```python
from build123d import *

# Parameters (mm, degrees)
SKETCH_1_W               = 40
SKETCH_1_H               = 65
SKETCH_1_R               = 12.5
EXTRUDE_1_DEPTH          = 2
CUT_EXTRUDE_1_DEPTH      = 39.369910086
CUT_EXTRUDE_1_DEPTH_BACK = 39.369910086
SKETCH_2_R               = 2.1
CHAMFER_2_SIZE           = 5


with BuildPart() as part:
    # 草图1 → 凸台-拉伸1 (new, symmetric)
    with BuildSketch(Plane.XY):
        Rectangle(SKETCH_1_W, SKETCH_1_H)
        Circle(SKETCH_1_R, mode=Mode.SUBTRACT)
    extrude(amount=EXTRUDE_1_DEPTH, both=True)

    # 草图2 → 切除-拉伸1 (cut, two sides: drawn at the far end of the back side and taken through both)
    with BuildSketch(Plane(origin=(0, 0, -2), x_dir=(-1, 0, 0), z_dir=(0, 0, -1)).offset(-CUT_EXTRUDE_1_DEPTH_BACK)):
        with Locations((-10, 22.5)):
            Circle(SKETCH_2_R)
        with Locations((10, 22.5)):
            Circle(SKETCH_2_R)
        with Locations((10, -22.5)):
            Circle(SKETCH_2_R)
        with Locations((-10, -22.5)):
            Circle(SKETCH_2_R)
    extrude(amount=CUT_EXTRUDE_1_DEPTH + CUT_EXTRUDE_1_DEPTH_BACK, mode=Mode.SUBTRACT)

    # 倒角2
    chamfer_2_edges = [part.edges().sort_by_distance(p)[0] for p in [
        (-20, 32.5, 0),
        (20, 32.5, 0),
        (20, -32.5, 0),
        (-20, -32.5, 0),
    ]]
    chamfer(chamfer_2_edges, length=CHAMFER_2_SIZE)


solid = part.part
```
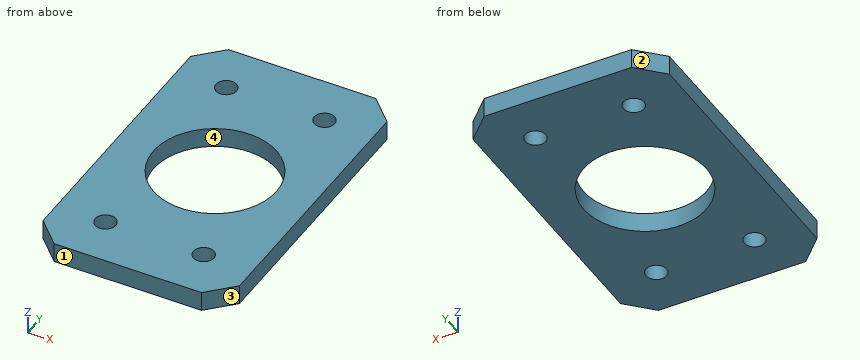
The model under review builds one solid part; all positions refer to its coordinate system, in mm. Face numbers are marked on the shaded views. Coordinates: 2 decimals unless noted, no trailing zeros. Write each loop counter-clockwise with the first axis right and the second up, starting at its lowest first coordinate (ties: lowest second). Pieces come first, ordered by that corner, then holes. Notation, with made-up numbers: (2.5, 75.5) - (54.5, 75.5) arc R30 ccw to (54.5, 100.5) - close; hole circle Ø6 at (33, 25). An arc over 180 degrees is marked (long way). Answer in a Markdown table with one row per item. Add a question column.
Q1. To check wall thickness, follow line 1 along X through (y, z) = (22.5, -0.5); line 2 along Y through (x, z) = (0, -0.95); line 3 along Y through (x, z) = (10, -0.15). State the ranges of each line that lie inside material, in increasing order. Write a range as from..to.
Q2. Consider section B-B on y = -22.5. Give the boundary of the cut face in (x, z), then the cut area to 3 significant figures.
Q3. Clearance check with a flat-ended pin moving along its axis: pin 1 (2.5 mm diameter, centred on x = 10, y = 22.5, fed in from -Z). State where the tip first meets the part, or that it passes through.
Q4. Consider section C-C on x = 0. Give the boundary of the cut face in (y, z), then the cut area to 3 significant figures.
Q5. Consider section D-D on y = 0. Give the boundary of the cut face in (x, z), then the cut area to 3 significant figures.
Q6. Draft analysis for pull direction X (two halves, no side actions). For the marked faces 1, 2, 3 and 4, state which applies: +X half, -X half, draft (parallel to the pull), parting line (faces both ways), or undercut.
Q7. Consider section A-A on x = 10. Give the boundary of the cut face in (y, z).
Answers below:
| question | item | result |
|---|---|---|
| 1 | line 1 | -20..-12.1, -7.9..7.9, 12.1..20 |
| 1 | line 2 | -32.5..-12.5, 12.5..32.5 |
| 1 | line 3 | -32.5..-24.6, -20.4..-7.5, 7.5..20.4, 24.6..32.5 |
| 2 | outline | (-20, -2) - (-12.1, -2) - (-12.1, 2) - (-20, 2) - close; (-7.9, -2) - (7.9, -2) - (7.9, 2) - (-7.9, 2) - close; (12.1, -2) - (20, -2) - (20, 2) - (12.1, 2) - close |
| 2 | area | 126 mm² |
| 3 | pin 1 | through |
| 4 | outline | (-32.5, -2) - (-12.5, -2) - (-12.5, 2) - (-32.5, 2) - close; (12.5, -2) - (32.5, -2) - (32.5, 2) - (12.5, 2) - close |
| 4 | area | 160 mm² |
| 5 | outline | (-20, -2) - (-12.5, -2) - (-12.5, 2) - (-20, 2) - close; (12.5, -2) - (20, -2) - (20, 2) - (12.5, 2) - close |
| 5 | area | 60.0 mm² |
| 6 | face 1 | draft |
| 6 | face 2 | -X half |
| 6 | face 3 | +X half |
| 6 | face 4 | undercut |
| 7 | outline | (-32.5, -2) - (-24.6, -2) - (-24.6, 2) - (-32.5, 2) - close; (-20.4, -2) - (-7.5, -2) - (-7.5, 2) - (-20.4, 2) - close; (7.5, -2) - (20.4, -2) - (20.4, 2) - (7.5, 2) - close; (24.6, -2) - (32.5, -2) - (32.5, 2) - (24.6, 2) - close |
